Geometry check sheet. Reference: the model listing, model coordinates, mm. Face numbers are marked on the shaded views. Give positions to 0.01 mm unless a question says otherwise; leave off trailing zeros. Write each loop counter-clockwise with the first axis right and the second up, starting at its lowest first coordinate (ties: lowest second). Pieces come first, ordered by that corner, then holes.
(1) Cross-section at A-A (y = 0). Record the boundary of the cut face in (x, z).
(2) Mould release check, pull along X, two halves, no side actions. Record for the marked faces 1, 2, 3 and 4: +X half, -X half, draft (parallel to the pull), parting line (faces both ways), or undercut.
(3) Cross-section at D-D (y = -12). Record the boundary of the cut face in (x, z), and give its area (3 significant figures).
(4) Cross-section at B-B (x = 0). Record the boundary of the cut face in (y, z), and give its area (3 significant figures).
(5) Thickness scan on line 1 along X through (y, z) = (46.5, 15.5); line 2 along X through (y, z) = (-23.5, 20); line 3 along X through (y, z) = (-19.5, 20.25). Record the ranges inside material, lowest first.
(6) Cross-section at C-C (z = 3.75). Record the boundary of the cut face in (x, y), and give its area (3 significant figures).
```python
from build123d import *

# Parameters (mm, degrees)
F0_W     = 200
F0_H     = 100
F0_R     = 35
F1_DEPTH = 25
F2_W     = 15
F2_H     = 100
F3_DEPTH = 10
F4_W     = 27.6011
F4_H     = 100
F5_DEPTH = 10


with BuildPart() as f1:
    # F0 (on Top) → F1 (new body)
    with BuildSketch(Plane.XY):
        Rectangle(F0_W, F0_H)
        Circle(F0_R, mode=Mode.SUBTRACT)
    extrude(amount=F1_DEPTH)

    # F2 (on face) → F3 (cut)
    with BuildSketch(Plane.XY.offset(25)):
        with Locations((-72.5, 0)):
            Rectangle(F2_W, F2_H)
    extrude(amount=-F3_DEPTH, mode=Mode.SUBTRACT)

    # F4 (on face) → F5 (cut)
    with BuildSketch(Plane.XY.offset(25)):
        with Locations((66.783089, 0)):
            Rectangle(F4_W, F4_H)
    extrude(amount=-F5_DEPTH, mode=Mode.SUBTRACT)


solid = f1.part
```
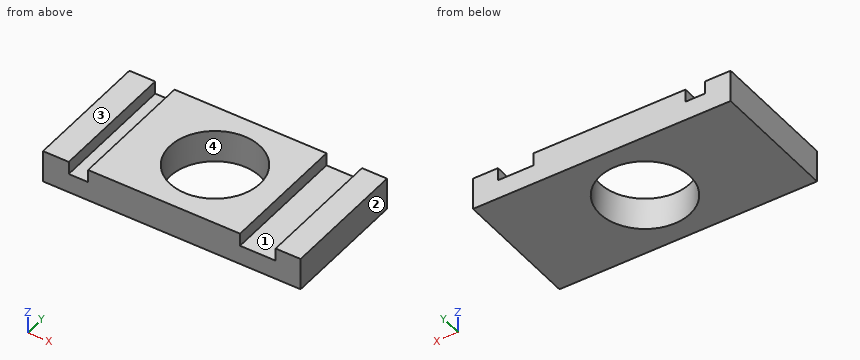
Reply:
1. outline: (-100, 0) - (-35, 0) - (-35, 25) - (-65, 25) - (-65, 15) - (-80, 15) - (-80, 25) - (-100, 25) - close; (35, 0) - (100, 0) - (100, 25) - (80.58, 25) - (80.58, 15) - (52.98, 15) - (52.98, 25) - (35, 25) - close
2. face 1: undercut
2. face 2: +X half
2. face 3: draft
2. face 4: undercut
3. outline: (-100, 0) - (-32.88, 0) - (-32.88, 25) - (-65, 25) - (-65, 15) - (-80, 15) - (-80, 25) - (-100, 25) - close; (32.88, 0) - (100, 0) - (100, 25) - (80.58, 25) - (80.58, 15) - (52.98, 15) - (52.98, 25) - (32.88, 25) - close
3. area: 2,930 mm2
4. outline: (-50, 0) - (-35, 0) - (-35, 25) - (-50, 25) - close; (35, 0) - (50, 0) - (50, 25) - (35, 25) - close
4. area: 750 mm2
5. line 1: x = -100 to -80, -65 to 52.98, 80.58 to 100
5. line 2: x = -100 to -80, -65 to -25.94, 25.94 to 52.98, 80.58 to 100
5. line 3: x = -100 to -80, -65 to -29.06, 29.06 to 52.98, 80.58 to 100
6. outline: (-100, -50) - (100, -50) - (100, 50) - (-100, 50) - close; hole circle Ø70 at (0, 0)
6. area: 16,200 mm2
